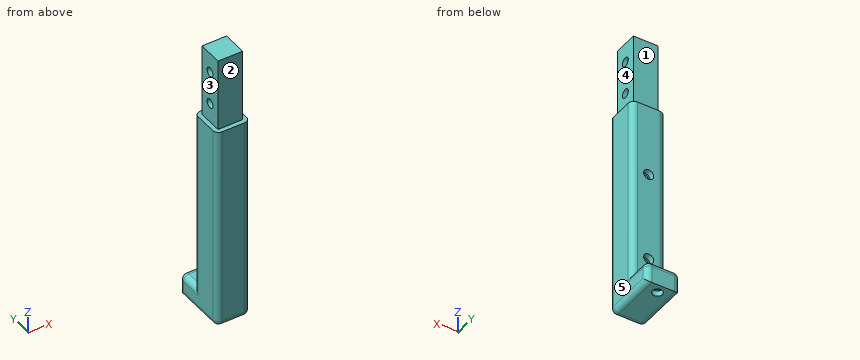
Autodesk Inventor part; units mm, degrees
ref_plane "YZ Plane" through (0, 0, 0) normal (1, 0, 0) x (0, 1, 0)
ref_plane "XZ Plane" through (0, 0, 0) normal (0, 1, 0) x (-1, 0, 0)
ref_plane "XY Plane" through (0, 0, 0) normal (0, 0, 1) x (1, 0, 0)
sketch "Sketch1" plane through (0, 0, 0) normal (0, 1, 0) x (-1, 0, 0)
  line L0 (15, 124.835) -> (-15, 124.835)
  line L1 (-15, 124.835) -> (-15, -124.835)
  line L2 (-15, -124.835) -> (15, -124.835)
  line L3 (15, -124.835) -> (15, 124.835)
  line L4 (15, 124.835) -> (-15, -124.835) construction
  line L5 (-15, 124.835) -> (15, -124.835) construction
  point P0 (0, 0)
  dimension "d0" = 30
  dimension "d1" = 249.67
extrude "Extrusion1" add sketch "Sketch1" along normal blind 30
sketch "Sketch2" plane through (0, 30, 0) normal (0, 1, 0) x (1, 0, 0)
  line L0 (15, 124.835) -> (-15, 124.835)
  line L1 (-15, 124.835) -> (-15, -124.835)
  line L2 (15, 124.835) -> (-15, 124.835)
  line L3 (-15, 124.835) -> (-15, 104.835)
  line L4 (-15, 104.835) -> (15, 104.835)
  line L5 (15, 104.835) -> (15, 124.835)
  point P0 (0, 0)
  dimension "d4" = 20
extrude "Extrusion2" add sketch "Sketch2" along normal blind 20
sketch "Sketch3" plane through (-15, 0, 124.835) normal (0, 0, 1) x (1, 0, 0)
  line L0 (0, 0) -> (30, 0)
  line L1 (30, 0) -> (30, 30)
  line L2 (0, 30) -> (30, 30)
  line L3 (0, 0) -> (0, 30)
  line L4 (4, 26) -> (26, 26)
  line L5 (26, 26) -> (26, 4)
  line L6 (26, 4) -> (4, 4)
  line L7 (4, 4) -> (4, 26)
  point P0 (15, 0)
  dimension "d7" = 4
extrude "Extrusion3" cut sketch "Sketch3" against normal blind 65
sketch "Sketch4" plane through (15, 0, -124.835) normal (0, 0, -1) x (-1, 0, 0)
  line L0 (0, 50) -> (30, 50)
  line L1 (30, 0) -> (30, 50)
  point P0 (15, 0)
  point P1 (15, 42)
  dimension "d10" = 8
  dimension "d11" = 15
hole "Hole1" at (0, 42, -124.835) direction (0, 0, 1) diameter 6 depth 10 tip angle 118 counterbore diameter 9 counterbore depth 5
sketch "Sketch5" plane through (11, 4, 124.835) normal (1, 0, 0) x (0, 0, -1)
  circle A0 centre (17.5, 11) radius 4
  circle A1 centre (47.5, 11) radius 4
  line L0 (65, 26) -> (65, -4)
  line L1 (0, 0) -> (0, 22)
  line L2 (0, 0) -> (65, 0)
  point P0 (124.835, -4)
  point P1 (65, 11)
  point P2 (0, 11)
  dimension "d19" = 8
  dimension "d20" = 8
  dimension "d21" = 30
  dimension "d23" = 17.5
extrude "Extrusion4" cut sketch "Sketch5" against normal through all
fillet "Fillet1" radius 5 12 edges at (15, 25, -124.835) (-15, 25, -124.835) (0, 0, -124.835) (15, 0, -32.5) (-15, 0, -32.5) (15, 30, -22.5) (-15, 30, -22.5) (15, 40, -104.835) (-15, 40, -104.835) (0, 50, -104.835) (15, 50, -114.835) (-15, 50, -114.835)
sketch "Sketch6" plane through (0, 30, 0) normal (0, 1, 0) x (1, 0, 0)
  line L0 (-10, 104.835) -> (10, 104.835)
  line L1 (-10, -59.835) -> (-10, 104.835)
  point P0 (0, 0)
  point P1 (0, 84.835)
  point P2 (0, 4.835)
  dimension "d28" = 20
  dimension "d36" = 100
  dimension "d37" = 10
  dimension "d38" = 10
hole "Hole2" at (0, 30, -4.835) at (0, 30, -84.835) direction (0, -1, 0) diameter 6 depth 10 tip angle 118 counterbore diameter 9 counterbore depth 5
properties part number "L" material "PCTG 20%"
Can you work these out from the model? Positions are in its coordinate system, mm. Face numbers are marked on the shaded views. A direction names the side the tool comes from. Round coordinates to 2 decimals unless told otherwise and drop trailing zeros. Loops run counter-clockwise (first coordinate to the right, second up) from the corner with the lowest first, then second, coordinate; pieces in that order, holes last. Notation, with made-up numbers: (26.25, -29.75) - (66.25, -29.75) arc R38 cw to (66.25, 8.25) - close; hole circle Ø9 at (72, 40.25). An arc over 180 degrees is marked (long way). Answer in a Markdown table with one row per item. Add a question column.
Q1. I want a section at D-D on z = 90. List the corners of the cut face in (x, y) for me, and give its area (3 significant figures).
Q2. I want a section at A-A on y = 15. List the corners of the cut face in (x, z) for me (3 decimals).
Q3. For pin 1 Ø11 at (y, z) = (10, 96.5) entering from -X; pin 2 Ø4.5 at (x, z) = (2, -83.5) entering from +Y; pin 3 Ø5 at (x, y) = (0, 42) entering from +Z (3 decimals), each with a flat end and sliding along its axis, tell me the tip position at first contact or that it passes through.
Q4. I want a section at B-B on z = 35.5. List the corners of the cut face in (x, y) for me, and give its area (3 significant figures).
Q5. Which directions (+Z, -Z, +X, -X, +Y, -Y) give clear straight access to the entire face, cutting with the end or side of a thin tool? Please do the marked faces 1, 2, 3, 4 and 5.
Q6. I want a section at C-C on y = 35. List the corners of the cut face in (x, z) for me (3 decimals), and give its area (3 significant figures).
Q7. I need wall thicknesses on L1, parallel to Z at x = 0, y = 27.25 (3 decimals); L2, parallel to Z at x = 0, y = 23.8 (3 decimals); L3, parallel to Z at x = 8, y = 43.5 (3 decimals). Which ranges of each line are inside material? Lowest first, please.
A:
| question | item | result |
|---|---|---|
| 1 | outline | (-11, 4) - (11, 4) - (11, 26) - (-11, 26) - close |
| 1 | area | 484 mm^2 |
| 2 | outline | (-15, -119.835) arc R5 ccw to (-10, -124.835) - (10, -124.835) arc R5 ccw to (15, -119.835) - (15, 59.835) - (11, 59.835) - (11, 73.335) - (-11, 73.335) - (-11, 59.835) - (-15, 59.835) - close; (-11, 81.335) - (11, 81.335) - (11, 103.335) - (-11, 103.335) - close; (-11, 111.335) - (11, 111.335) - (11, 124.835) - (-11, 124.835) - close |
| 3 | pin 1 | x = -11 |
| 3 | pin 2 | y = 30 |
| 3 | pin 3 | z = -104.835 |
| 4 | outline | (-15, 5) arc R5 ccw to (-10, 0) - (10, 0) arc R5 ccw to (15, 5) - (15, 25) arc R5 ccw to (10, 30) - (-10, 30) arc R5 ccw to (-15, 25) - close |
| 4 | area | 879 mm^2 |
| 5 | face 1 | +Z, +X, -X, +Y |
| 5 | face 2 | +Z, +X, -X, -Y |
| 5 | face 3 | +Z, -X, +Y, -Y |
| 5 | face 4 | +Z, +X, +Y, -Y |
| 5 | face 5 | +Z, -Z, +X, +Y, -Y |
| 6 | outline | (-15, -119.835) arc R5 ccw to (-10, -124.835) - (10, -124.835) arc R5 ccw to (15, -119.835) - (15, -109.835) arc R5 ccw to (10, -104.835) - (-10, -104.835) arc R5 ccw to (-15, -109.835) - close |
| 6 | area | 579 mm^2 |
| 7 | L1 | -124.835 to -89.335, -80.335 to -9.335, -0.335 to 59.835 |
| 7 | L2 | -124.835 to -87.835, -81.835 to -7.835, -1.835 to 124.835 |
| 7 | L3 | -124.835 to -104.835 |
